Could you check a few things on this model? Use its own coordinates, in mm. Face numbers are marked on the shaded views. A direction names the side the tool comes from. Give positions to 0.01 mm unless a question says otherwise; leave off trailing zeros. Write each loop counter-clockwise with the first axis right and the second up, starting at its lowest first coordinate (ties: lowest second). Pieces come first, ordered by that corner, then holes. Notation, with made-up numbers: (85, 42.25) - (143, 42.25) arc R33 ccw to (143, 79.25) - close; hole circle Ø6 at (60.25, 82.25). An arc over 180 degrees is marked (long way). Answer in a Markdown table with one row per item.
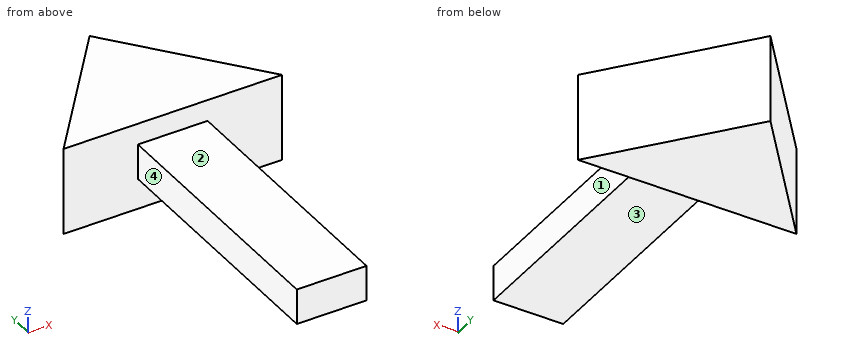
from build123d import *

# Parameters (mm, degrees)
F1_DEPTH = 25.4
F2_W     = 75.767048
F2_H     = 10.304318
F3_DEPTH = 10.12838


with BuildPart() as f1:
    # F0 (on Top) → F1 (new body)
    with BuildSketch(Plane.XY):
        Polygon((31.75, 0), (0, 39.655737), (-31.75, 0), align=None)
    extrude(amount=F1_DEPTH)

    # F2 (on Right) → F3 (join, symmetric)
    with BuildSketch(Plane.YZ):
        with Locations((-37.883524, 14.042159)):
            Rectangle(F2_W, F2_H)
    extrude(amount=F3_DEPTH, both=True)


solid = f1.part
1) On a 3-axis mill with a long thin cutter (end or side, diameter ignored), from which of +Z, -Z, +X, -X, +Y, -Y can I reach the whole of each face in a straight line? I mean the marked faces 1, 2, 3 and 4. Say none if no direction works.
Check values:
| item | result |
|---|---|
| face 1 | +Z, -Z, +X, -Y |
| face 2 | +Z, +X, -X, -Y |
| face 3 | -Z, +X, -X, -Y |
| face 4 | +Z, -Z, -X, -Y |
2) If I drill on line 1 (X direction, y = -59, z = 16); line 2 (Z direction, x = 1, y = -24.5); line 3 (Y direction, x = -15.5, z = 13.5), over which ranges is the centre line in solid material (lowest first)?
Check values:
| item | result |
|---|---|
| line 1 | x = -10.13 to 10.13 |
| line 2 | z = 8.89 to 19.19 |
| line 3 | y = 0 to 20.3 |
3) Imagine slicing it at D-D (x = 8.5). List the corners of the cut face in (y, z) for me, then the cut area to 3 significant figures.
Check values:
| item | result |
|---|---|
| outline | (-75.77, 8.89) - (0, 8.89) - (0, 0) - (29.04, 0) - (29.04, 25.4) - (0, 25.4) - (0, 19.19) - (-75.77, 19.19) - close |
| area | 1,520 mm2 |
4) Will these pins go through, and if not, where does the flat tip stop? P1, Ø10, axis at y = -20.5, z = 18, coming from the +X side; P2, Ø16, axis at x = 0.5, y = -35, coming from the +Z side; P3, Ø22.5, axis at x = 0, y = -27, coming from the -Z side; P4, Ø6, axis at y = -60, z = 4, coming from the -X side.
Check values:
| item | result |
|---|---|
| P1 | stops at x = 10.13 |
| P2 | stops at z = 19.19 |
| P3 | stops at z = 8.89 |
| P4 | passes through |
5) Imagine slicing it at C-C (y = -54.5). List the corners of the cut face in (x, z) for me, then the cut area to 3 significant figures.
Check values:
| item | result |
|---|---|
| outline | (-10.13, 8.89) - (10.13, 8.89) - (10.13, 19.19) - (-10.13, 19.19) - close |
| area | 209 mm2 |
6) Imagine slicing it at A-A (z = 12.75). List the corners of the cut face in (x, y) for me.
Check values:
| item | result |
|---|---|
| outline | (-31.75, 0) - (-10.13, 0) - (-10.13, -75.77) - (10.13, -75.77) - (10.13, 0) - (31.75, 0) - (0, 39.66) - close |
7) Imagine slicing it at B-B (x = -5). List the corners of the cut face in (y, z) for me.
Check values:
| item | result |
|---|---|
| outline | (-75.77, 8.89) - (0, 8.89) - (0, 0) - (33.41, 0) - (33.41, 25.4) - (0, 25.4) - (0, 19.19) - (-75.77, 19.19) - close |
